Check sheet for the drawn part. Datum: minimum x, y, z corner. Units: mm. A direction names the side the tool comes from. Give positions to 0.01 mm unless a question says otherwise; leave off trailing zeros. Write each loop counter-clockwise with the first axis right and the second up, starting at its lowest first coordinate (ties: lowest second). Pieces come first, ordered by that corner, then holes. Notation, with made-up numbers: (53, -4.75) - (77, -4.75) arc R30 ccw to (77, 19.25) - close; hole circle Ø8 at (86.5, -22). An arc over 180 degrees is marked (long way). Answer as a JSON object with one key per item and string values. Group by question number.
Item 1: Scan lines: line 1 along Z through (x, y) = (6.35, 1.5); line 2 along X through (y, z) = (33, 6); line 3 along Y through (x, z) = (14.5, 12). Record each from-to range of solid material in increasing order. Write a range as [from, to].
Item 2: Sectioned sample at B-B, the plane y = 44. Record the boundary of the cut face in (x, z).
Item 3: Go/stop test with flat-tipped pins: pin 1 (3 mm diameter, centred on x = 6.35, z = 15.875, fed in from +Y); pin 2 (1.5 mm diameter, centred on x = 16, z = 11.5, fed in from +Y); pin 3 (2 mm diameter, centred on y = 29, z = 19.5, fed in from -X); pin 4 (10 mm diameter, centred on x = 32.5, z = 9.5, fed in from +Y). Record where each tip stops, or that it passes through.
Item 4: Sectioned sample at A-A, the plane x = 6.35. Record the boundary of the cut face in (y, z), and give its area (3 significant figures).
Item 5: Tool access check on the marked faces 1 and 2. Record the directions out of +Z, -Z, +X, -X, +Y, -Y that give a thin tool (end or side, any length) a straight path to the whole face; none if there is none.
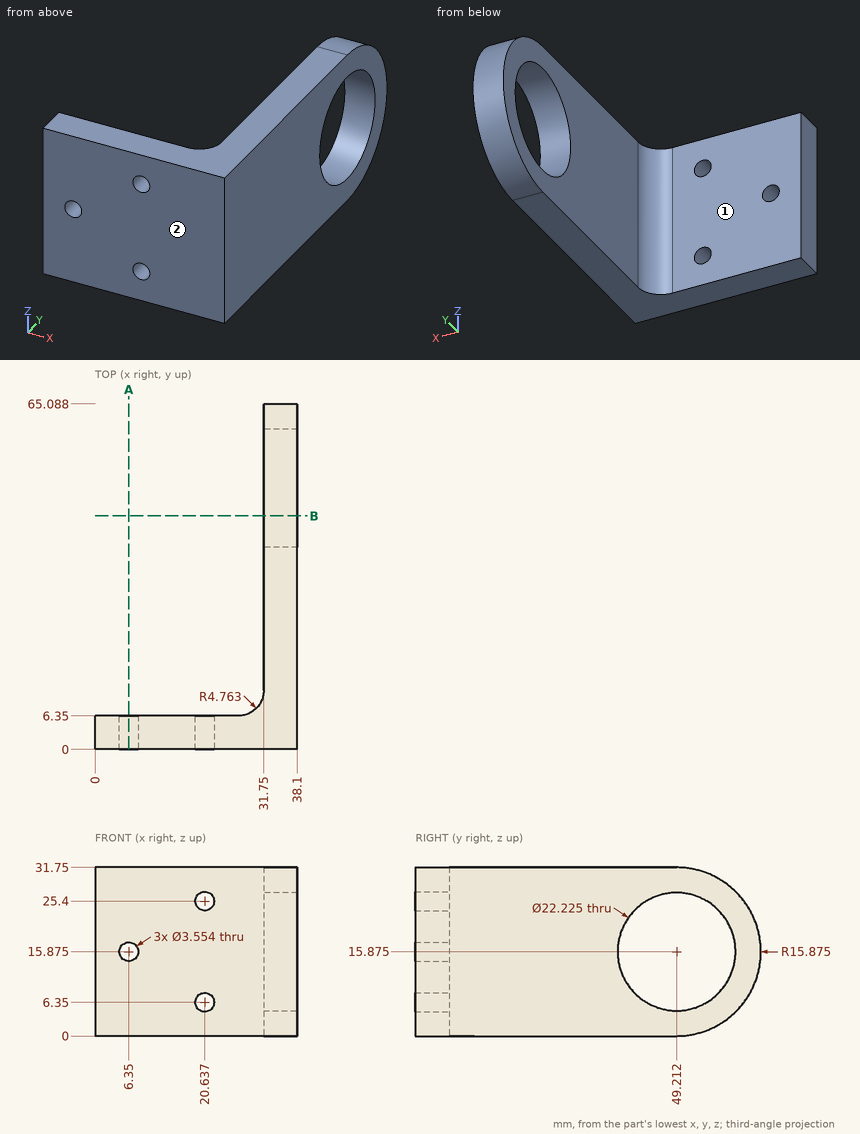
Geometry check:
{
 "1": {"line 1": "[0, 14.1], [17.65, 31.75]", "line 2": "[31.75, 38.1]", "line 3": "[0, 6.35]"},
 "2": {"outline": "(31.75, 0) - (38.1, 0) - (38.1, 6.06) - (31.75, 6.06) - close; (31.75, 25.69) - (38.1, 25.69) - (38.1, 31.75) - (31.75, 31.75) - close"},
 "3": {"pin 1": "through", "pin 2": "y = 6.35", "pin 3": "x = 31.75", "pin 4": "y = 65.03"},
 "4": {"outline": "(0, 0) - (6.35, 0) - (6.35, 14.1) - (0, 14.1) - close; (0, 17.65) - (6.35, 17.65) - (6.35, 31.75) - (0, 31.75) - close", "area": "179 mm^2"},
 "5": {"face 1": "+Z, -Z, -X, +Y", "face 2": "+Z, -Z, +X, -X, -Y"}
}
